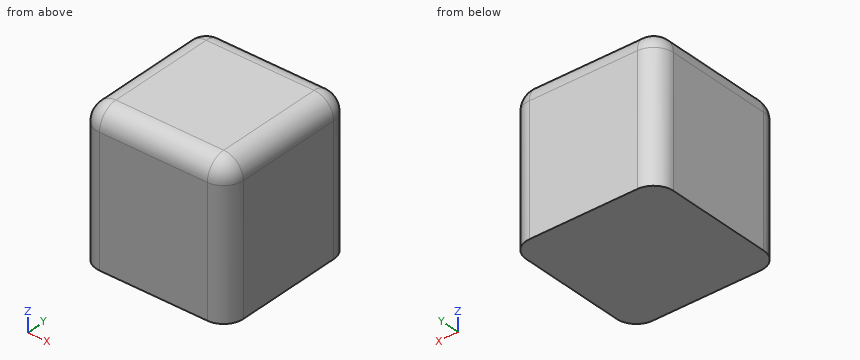
from build123d import *

# Parameters (mm, degrees)
F1_W     = 38.1
F1_H     = 38.1
F2_DEPTH = 19.05
F3_R     = 5.08


with BuildPart() as f2:
    # F1 (on face) → F2 (new body, symmetric)
    with BuildSketch(Plane.XY):
        Rectangle(F1_W, F1_H)
    extrude(amount=F2_DEPTH, both=True)

    # F3
    f3_edges = [f2.edges().sort_by_distance(p)[0] for p in [
        (0, -19.05, 19.05),
        (19.05, 0, 19.05),
        (0, 19.05, 19.05),
        (-19.05, 0, 19.05),
        (19.05, -19.05, 0),
        (-19.05, -19.05, 0),
        (19.05, 19.05, 0),
        (-19.05, 19.05, 0),
    ]]
    fillet(f3_edges, radius=F3_R)


solid = f2.part
Build history of the part. All positions in model axes, mm. Round coordinates to 2 decimals unless told otherwise and drop trailing zeros. Loops run counter-clockwise (first coordinate to the right, second up) from the corner with the lowest first, then second, coordinate; pieces in that order, holes last. Notation, with made-up numbers: (45, 11) -> (92, 11) arc R28 cw to (92, 49) -> close; hole circle Ø4 at (42.25, 54.5). An arc over 180 degrees is marked (long way). One line per item, written item: value. Start each with the question number.
Q1. Drop flat-ended pins along their axis: pin 1 Ø4 at (y, z) = (-14.5, -7.5) entering from +X; pin 2 Ø1 at (x, z) = (15, 7.5) entering from +Y. Give the stop position or say it passes through.
Q2. Cut at B-B on x = 15. List the corners of the cut face in (y, z).
Q3. Cut at A-A on z = 7.5. List the corners of the cut face in (x, y).
Q4. Cut at D-D on z = 15.5. List the corners of the cut face in (x, y), plus the area to 3 significant figures.
Q5. Probe line 1 along Y through (x, z) = (-7, 17); line 2 along Y through (x, z) = (-16.5, 13.5). List the from-to ranges inside material, lowest first.
Q6. Cut at C-C on y = -16. List the corners of the cut face in (x, z).
Computed:
1. pin 1: x = 19.05
1. pin 2: y = 19.02
2. outline: (-18.94, -19.05) -> (18.94, -19.05) -> (18.94, 13.97) arc R4.97 ccw to (13.97, 18.94) -> (-13.97, 18.94) arc R4.97 ccw to (-18.94, 13.97) -> close
3. outline: (-19.05, -13.97) arc R5.08 ccw to (-13.97, -19.05) -> (13.97, -19.05) arc R5.08 ccw to (19.05, -13.97) -> (19.05, 13.97) arc R5.08 ccw to (13.97, 19.05) -> (-13.97, 19.05) arc R5.08 ccw to (-19.05, 13.97) -> close
4. outline: (-18.81, -13.97) arc R4.84 ccw to (-13.97, -18.81) -> (13.97, -18.81) arc R4.84 ccw to (18.81, -13.97) -> (18.81, 13.97) arc R4.84 ccw to (13.97, 18.81) -> (-13.97, 18.81) arc R4.84 ccw to (-18.81, 13.97) -> close
4. area: 1,400 mm²
5. line 1: -18.05 to 18.05
5. line 2: -18.38 to 18.38
6. outline: (-18.63, -19.05) -> (18.63, -19.05) -> (18.63, 13.97) arc R4.66 ccw to (13.97, 18.63) -> (-13.97, 18.63) arc R4.66 ccw to (-18.63, 13.97) -> close
